Design review of the part shown in the three views and the two pictorial views. Dimensions are in mm from the part's minimum x, y and z. A direction names the side the tool comes from. Round coordinates to 2 decimals unless told otherwise and drop trailing zeros. Write each loop counter-clockwise with the first axis right and the second up, starting at its lowest first coordinate (ties: lowest second). Pieces come first, ordered by that corner, then holes. Notation, with made-up numbers: (-36, -27.75) -> (-4, -27.75) arc R21 cw to (-4, -18.75) -> close; hole circle Ø5 at (4, 32.25). An arc over 180 degrees is marked (long way). Answer as a JSON object with one key per item and string values. Group by question number.
1) Machinability: for the marked faces 1, 2, 3, 4 and 5, which of the approach directions +Z, -Z, +X, -X, +Y, -Y give a long, thin tool a straight path to every point of the face, cutting with its end or side? Answer none if there is none.
2) To check wall thickness, follow probe 1 along Z at (x, y) = (5.5, 5.75); probe 2 along X at (y, z) = (11, 16); probe 3 along Z at (x, y) = (3.25, 11.25). State the ranges of each line that lie inside material, in increasing order. Write a range as [from, to].
3) We need section C-C, the plane z = 24.75. Write out the cut boundary in (x, y).
4) We need section B-B, the plane y = 11.25. Write out the cut boundary in (x, z), then the cut area to 3 significant figures.
5) We need section A-A, the plane x = 11.25. Write out the cut boundary in (y, z).
6) Insertion check: pin 1 Ø1.6 at (x, z) = (11, 28) entering from -Y; pin 2 Ø0.6 at (y, z) = (11, 29) entering from +X; pin 3 Ø1.5 at (x, z) = (12.5, 16) entering from +Y. Each pin has a flat end and moves straight along its axis. Give the tip position at first contact, or say it passes through.
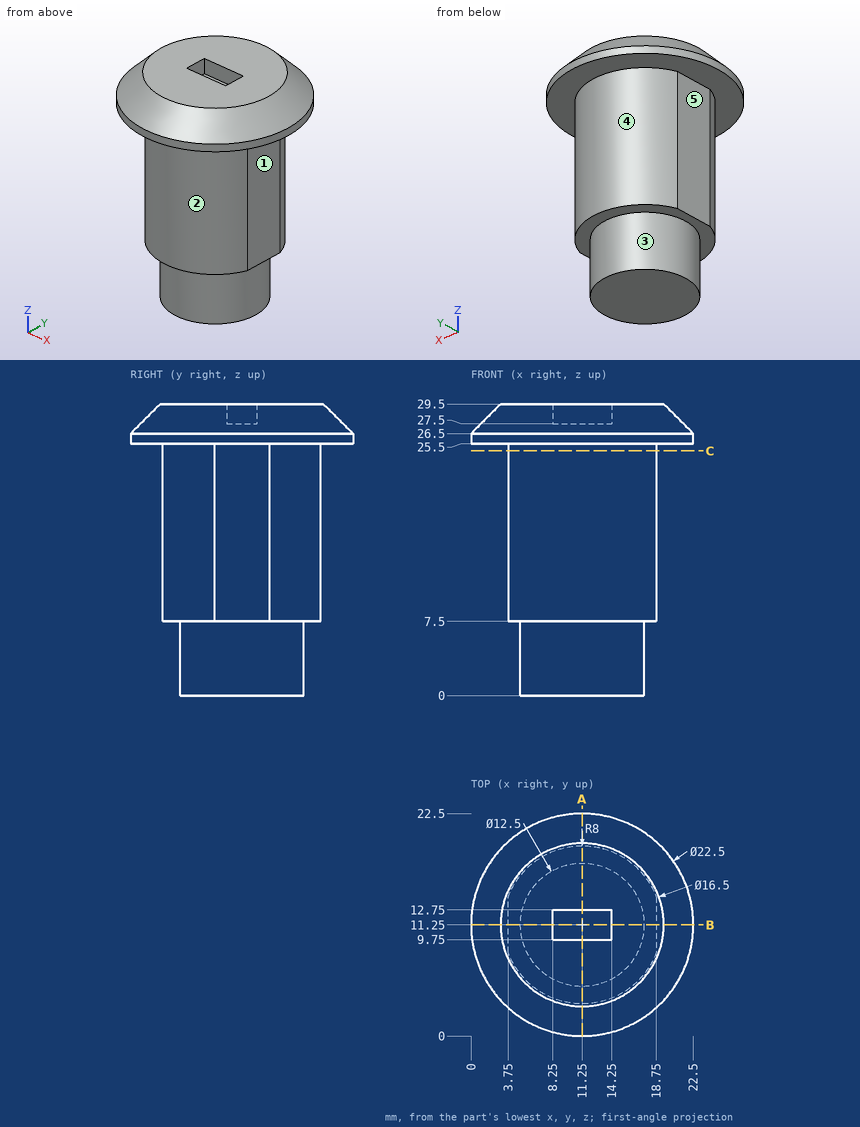
Here are the results:
{
 "1": {"face 1": "-Z, +X, +Y, -Y", "face 2": "-Z, -Y", "face 3": "-Z", "face 4": "-Z, +Y", "face 5": "-Z, -X, +Y, -Y"},
 "2": {"probe 1": "z = [7.5, 29.5]", "probe 2": "x = [3.75, 18.75]", "probe 3": "z = [25.5, 29.5]"},
 "3": {"outline": "(3.75, 8.47) arc R8 ccw to (18.75, 8.47) -> (18.75, 14.03) arc R8 ccw to (3.75, 14.03) -> close"},
 "4": {"outline": "(0, 25.5) -> (3.75, 25.5) -> (3.75, 7.5) -> (5, 7.5) -> (5, 0) -> (17.5, 0) -> (17.5, 7.5) -> (18.75, 7.5) -> (18.75, 25.5) -> (22.5, 25.5) -> (22.5, 26.5) -> (19.5, 29.5) -> (14.25, 29.5) -> (14.25, 27.5) -> (8.25, 27.5) -> (8.25, 29.5) -> (3, 29.5) -> (0, 26.5) -> close", "area": "433 mm^2"},
 "5": {"outline": "(0, 25.5) -> (3.25, 25.5) -> (3.25, 7.5) -> (5, 7.5) -> (5, 0) -> (17.5, 0) -> (17.5, 7.5) -> (19.25, 7.5) -> (19.25, 25.5) -> (22.5, 25.5) -> (22.5, 26.5) -> (19.5, 29.5) -> (12.75, 29.5) -> (12.75, 27.5) -> (9.75, 27.5) -> (9.75, 29.5) -> (3, 29.5) -> (0, 26.5) -> close"},
 "6": {"pin 1": "stops at y = 0.7", "pin 2": "stops at x = 20.3", "pin 3": "stops at y = 19.23"}
}
